Check sheet for the modelled part. Datum: model origin and axes. Units: mm. Face numbers are marked on the shaded views. Round coordinates to 2 decimals unless told otherwise and drop trailing zeros. Write each loop counter-clockwise with the first axis right and the second up, starting at its lowest first coordinate (ties: lowest second). Pieces come first, ordered by that corner, then holes. Notation, with made-up numbers: (6, 14.5) -> (13, 14.5) arc R7 ccw to (13, 21.5) -> close; hole circle Ø9 at (49, 30). An arc over 180 degrees is marked (long way). One line per item, written item: value. Start each with the question number.
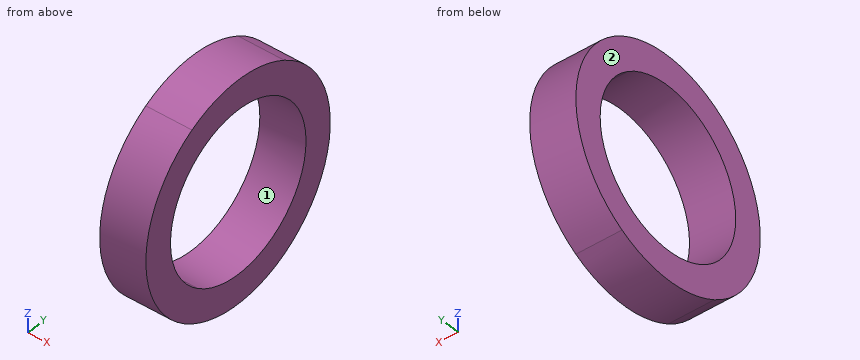
```python
from build123d import *
from build123d.topology import SkipClean

# Parameters (mm, degrees)
SKETCH1_W           = 200
SKETCH1_H           = 200
BOSS_EXTRUDE1_DEPTH = 30
SKETCH4_W           = 175
SKETCH4_H           = 175
CUT_EXTRUDE1_DEPTH  = 30
SKETCH7_R           = 4
CUT_EXTRUDE2_DEPTH  = 210
SKETCH10_W          = 6.040230253
SKETCH10_H          = 30
BOSS_EXTRUDE2_DEPTH = 20
SKETCH11_W          = 10
SKETCH11_H          = 30
BOSS_EXTRUDE3_DEPTH = 20
CUT_EXTRUDE3_START  = -231
SKETCH12_R          = 4
CUT_EXTRUDE3_DEPTH  = 231
SKETCH13_R          = 4
CUT_EXTRUDE5_DEPTH  = 231
SKETCH14_R          = 4
CUT_EXTRUDE6_DEPTH  = 250.5
SKETCH15_R          = 30
SKETCH15_R_2        = 22
BOSS_EXTRUDE5_DEPTH = 201
SKETCH17_R          = 22
CUT_EXTRUDE7_DEPTH  = 201
SKETCH21_W          = 9.5
SKETCH21_H          = 28.855904386
BOSS_EXTRUDE6_DEPTH = 26
SKETCH22_W          = 9.5
SKETCH22_H          = 6.040230253
CUT_EXTRUDE10_DEPTH = 49
SKETCH23_W          = 10.008922512
SKETCH23_H          = 28.855904386
BOSS_EXTRUDE7_DEPTH = 21
SKETCH24_W          = 9.5
SKETCH24_H          = 1.144095614
CUT_EXTRUDE11_DEPTH = 27
SKETCH26_W          = 0.50137975
SKETCH26_H          = 20.893624798
CUT_EXTRUDE12_DEPTH = 35
SKETCH27_R          = 49.192783102
CUT_EXTRUDE13_DEPTH = 175
SKETCH28_R          = 41.209023923
CUT_EXTRUDE14_DEPTH = 175
CUT_EXTRUDE15_START = -220
CUT_EXTRUDE15_DEPTH = 220
SKETCH33_R          = 22
CUT_EXTRUDE16_DEPTH = 220
SKETCH34_W          = 15.88682826
SKETCH34_H          = 39.259510286
CUT_EXTRUDE17_DEPTH = 14
SKETCH35_R          = 61.810225576
CUT_EXTRUDE18_DEPTH = 218


# Read off the part's stored shape, not the designer's step: Cut-Extrude15
with BuildPart() as part:
    # Sketch1 → Boss-Extrude1 (new body)
    with BuildSketch(Plane(origin=(0, 0, 0), x_dir=(1, 0, 0), z_dir=(0, 1, 0))):
        Rectangle(SKETCH1_W, SKETCH1_H)
    extrude(amount=BOSS_EXTRUDE1_DEPTH)

    # Sketch4 → Cut-Extrude1 (cut)
    with BuildSketch(Plane(origin=(0, 30, 0), x_dir=(1, 0, 0), z_dir=(0, 1, 0))):
        Rectangle(SKETCH4_W, SKETCH4_H)
    extrude(amount=-CUT_EXTRUDE1_DEPTH, mode=Mode.SUBTRACT)

    # Sketch7 → Cut-Extrude2 (cut)
    with BuildSketch(Plane.ZY.offset(100)):
        with Locations((0, 15)):
            Circle(SKETCH7_R)
    extrude(amount=-CUT_EXTRUDE2_DEPTH, mode=Mode.SUBTRACT)

    # Sketch10 → Boss-Extrude2 (add)
    with BuildSketch(Plane.ZY.offset(100)):
        with Locations((-11.64671233, 15)):
            Rectangle(SKETCH10_W, SKETCH10_H)
    extrude(amount=BOSS_EXTRUDE2_DEPTH)

    # Sketch11 → Boss-Extrude3 (add)
    with BuildSketch(Plane.XY.offset(-8.626597203)):
        with Locations((-115, 15)):
            Rectangle(SKETCH11_W, SKETCH11_H)
    extrude(amount=BOSS_EXTRUDE3_DEPTH)

    # Sketch12 → Cut-Extrude3 (cut)
    with BuildSketch(Plane(origin=(100, 0, 0), x_dir=(0, 0, -1), z_dir=(1, 0, 0)).offset(CUT_EXTRUDE3_START)):
        with Locations(Location((0, 15, 0), (0, 0, 180))):
            Circle(SKETCH12_R)
    extrude(amount=CUT_EXTRUDE3_DEPTH, mode=Mode.SUBTRACT)

    # Sketch13 → Cut-Extrude5 (cut)
    with BuildSketch(Plane(origin=(0, 30, 0), x_dir=(1, 0, 0), z_dir=(0, 1, 0))):
        with Locations(Location((-93.69452155, -93.045501349, 0), (0, 0, 270))):
            Circle(SKETCH13_R)
    extrude(amount=-CUT_EXTRUDE5_DEPTH, mode=Mode.SUBTRACT)

    # Sketch14 → Cut-Extrude6 (cut)
    with BuildSketch(Plane.XY.offset(100)):
        with Locations((0, 13.614739596)):
            Circle(SKETCH14_R)
    extrude(amount=-CUT_EXTRUDE6_DEPTH, mode=Mode.SUBTRACT)

    # Sketch15 → Boss-Extrude5 (add)
    with BuildSketch(Plane(origin=(100, 0, 0), x_dir=(0, 0, -1), z_dir=(1, 0, 0))):
        with Locations((0, 15)):
            Circle(SKETCH15_R)
        with Locations((0, 15)):
            Circle(SKETCH15_R_2, mode=Mode.SUBTRACT)
    extrude(amount=-BOSS_EXTRUDE5_DEPTH)

    # Sketch17 → Cut-Extrude7 (cut)
    with BuildSketch(Plane(origin=(100, 0, 0), x_dir=(0, 0, -1), z_dir=(1, 0, 0))):
        with Locations((0.074377339, 15.100772812)):
            Circle(SKETCH17_R)
    extrude(amount=-CUT_EXTRUDE7_DEPTH, mode=Mode.SUBTRACT)


with BuildPart() as cut_extrude7_piece_1:
    # of the separate pieces the step leaves, piece 1, a body of its own (cut_extrude7_pieces)
    add(part.part.solids().sort_by_distance((-100, 0, -100))[0])



with BuildPart() as cut_extrude7_piece_2:
    # of the separate pieces the step leaves, piece 2, a body of its own (cut_extrude7_pieces)
    add(part.part.solids().sort_by_distance((-101, 0, -14.666827456))[0])

    # Sketch21 → Boss-Extrude6 (add)
    with BuildSketch(Plane(origin=(0, 0, -14.666827456), x_dir=(-1, 0, 0), z_dir=(0, 0, -1))):
        with Locations((115.25, 15.572047807)):
            Rectangle(SKETCH21_W, SKETCH21_H)
    extrude(amount=BOSS_EXTRUDE6_DEPTH)

    # Sketch22 → Cut-Extrude10 (cut)
    with BuildSketch(Plane(origin=(0, 30, 0), x_dir=(1, 0, 0), z_dir=(0, 1, 0))):
        with Locations((-105.75, 11.64671233)):
            Rectangle(SKETCH22_W, SKETCH22_H)
    extrude(amount=-CUT_EXTRUDE10_DEPTH, mode=Mode.SUBTRACT)


with BuildPart() as cut_extrude7_piece_1_1:
    add(cut_extrude7_piece_1.part)

    add(cut_extrude7_piece_2.part)  # Boss-Extrude7 merges Cut-Extrude7 piece 2
    # Sketch23 → Boss-Extrude7 (add)
    with BuildSketch(Plane(origin=(-110.5, 0, 0), x_dir=(0, 0, -1), z_dir=(1, 0, 0))):
        with Locations((35.6623662, 15.572047807)):
            Rectangle(SKETCH23_W, SKETCH23_H)
    extrude(amount=BOSS_EXTRUDE7_DEPTH)

    # Sketch24 → Cut-Extrude11 (cut)
    with BuildSketch(Plane(origin=(0, 0, -14.666827456), x_dir=(-1, 0, 0), z_dir=(0, 0, -1))):
        with Locations((115.25, 0.572047807)):
            Rectangle(SKETCH24_W, SKETCH24_H)
    extrude(amount=-CUT_EXTRUDE11_DEPTH, mode=Mode.SUBTRACT)

    # Sketch26 → Cut-Extrude12 (cut)
    with BuildSketch(Plane.XZ):
        with Locations((-110.249310125, 1.820215196)):
            Rectangle(SKETCH26_W, SKETCH26_H)
    extrude(amount=-CUT_EXTRUDE12_DEPTH, mode=Mode.SUBTRACT)

    # Sketch27 → Cut-Extrude13 (cut)
    with BuildSketch(Plane(origin=(-87.5, 0, 0), x_dir=(0, 0, -1), z_dir=(1, 0, 0))):
        with Locations((-31.916352411, 15.376133278)):
            Circle(SKETCH27_R)
    extrude(amount=CUT_EXTRUDE13_DEPTH, mode=Mode.SUBTRACT)

    # Sketch28 → Cut-Extrude14 (cut)
    with BuildSketch(Plane(origin=(-87.5, 0, 0), x_dir=(0, 0, -1), z_dir=(1, 0, 0))):
        with Locations((37.762434774, 15.494435184)):
            Circle(SKETCH28_R)
    extrude(amount=CUT_EXTRUDE14_DEPTH, mode=Mode.SUBTRACT)

    # Cut-Extrude15 outline → Cut-Extrude15 (cut)
    with SkipClean():  # the faces are left unmerged after this step: merging them gives an invalid solid
        with BuildSketch(Plane(origin=(100, 0, 0), x_dir=(0, 0, -1), z_dir=(1, 0, 0)).offset(CUT_EXTRUDE15_START)):
            with BuildLine():
                ThreePointArc((25.980762114, 30), (30, 15), (25.980762114, 0))
                Line((25.980762114, 0), (100, 0))
                Line((100, 0), (100, 30))
                Line((100, 30), (25.980762114, 30))
            make_face()
            with BuildLine():
                ThreePointArc((-25.980762114, 0), (-30, 15), (-25.980762114, 30))
                Line((-25.980762114, 30), (-100, 30))
                Line((-100, 30), (-100, 0))
                Line((-100, 0), (-25.980762114, 0))
            make_face()
        extrude(amount=CUT_EXTRUDE15_DEPTH, mode=Mode.SUBTRACT)

    # Sketch33 → Cut-Extrude16 (cut)
    with SkipClean():  # the faces are left unmerged after this step: merging them gives an invalid solid
        with BuildSketch(Plane(origin=(100, 0, 0), x_dir=(0, 0, -1), z_dir=(1, 0, 0))):
            with Locations((0, 15)):
                Circle(SKETCH33_R)
        extrude(amount=-CUT_EXTRUDE16_DEPTH, mode=Mode.SUBTRACT)

    # Sketch34 → Cut-Extrude17 (cut)
    with SkipClean():  # the faces are left unmerged after this step: merging them gives an invalid solid
        with BuildSketch(Plane.ZY.offset(120)):
            with Locations((-24.036891069, 10.370244857)):
                Rectangle(SKETCH34_W, SKETCH34_H)
        extrude(amount=-CUT_EXTRUDE17_DEPTH, mode=Mode.SUBTRACT)

    # Sketch35 → Cut-Extrude18 (cut)
    with BuildSketch(Plane.ZY.offset(-87.5)):
        with Locations((-0.860757222, 19.909168714)):
            Circle(SKETCH35_R)
    extrude(amount=CUT_EXTRUDE18_DEPTH, mode=Mode.SUBTRACT)


solid = cut_extrude7_piece_1_1.part
```
1. Material ranges on probe 1 along Z at (x, y) = (93, 9); probe 2 along Z at (x, y) = (98.75, 24.5); probe 3 along Y at (x, z) = (90.5, 19), recorded low to high.
2. Cross-section at B-B (z = -20.5). Record the cut outline in (x, y).
3. Release check for a two-part mould opening along Y. For the marked faces 1 and 2 record: +Y half, -Y half, draft (parallel to the pull), parting line (faces both ways), or undercut.
4. Cross-section at C-C (y = 20). Record the cut outline in (x, z), plus the area to 3 significant figures.
5. Depth check by flat-ended pin: pin 1 Ø5 at (x, y) = (93.5, -2.5) entering from -Z; pin 2 Ø4 at (x, y) = (93, 21.5) entering from +Z; pin 3 Ø6 at (x, z) = (96, -7.5) entering from -Y. Enter the tip coordinate at first touch or a pass-through.
Working result:
1. probe 1: z = -29.39 to -21.21, 21.17 to 29.39
1. probe 2: z = -28.46 to -19.97, 19.84 to 28.46
1. probe 3: y = -8.22 to 3.91, 26.09 to 38.22
2. outline: (87.5, -6.9) -> (100, -6.9) -> (100, 6.93) -> (87.5, 6.93) -> close; (87.5, 23.27) -> (100, 23.27) -> (100, 36.9) -> (87.5, 36.9) -> close
3. face 1: undercut
3. face 2: draft
4. outline: (87.5, -29.58) -> (100, -29.58) -> (100, -21.52) -> (87.5, -21.52) -> close; (87.5, 21.42) -> (100, 21.42) -> (100, 29.58) -> (87.5, 29.58) -> close
4. area: 203 mm^2
5. pin 1: stops at z = -25.98
5. pin 2: stops at z = 29.66
5. pin 3: stops at y = -14.66
